```python
from build123d import *

# Parameters (mm, degrees)
F2_R     = 6.940355
F3_DEPTH = 279.4
F4_DEPTH = 25.4


with BuildPart() as f1:
    # F0 (on Front) → F1 (revolve)
    with BuildSketch(Plane.XZ):
        Polygon((0, -12.7), (0, 0), (53.81389, 53.949098), (49.866706, 57.886391), (-4.610259, 3.272552), (-12.603007, 2.86432), (-12.603007, -12.7), align=None)
    revolve(axis=Axis((-12.603007, 0, -4.91784), (0, 0, 1)))

    # F2 (on Top) → F3 (cut)
    with BuildSketch(Plane.XY):
        with Locations((-12.676277, 0)):
            Circle(F2_R)
    extrude(amount=-F3_DEPTH, mode=Mode.SUBTRACT)

    # F2 (on Top) → F4 (cut)
    with BuildSketch(Plane.XY):
        with Locations((-12.676277, 0)):
            Circle(F2_R)
    extrude(amount=F4_DEPTH, mode=Mode.SUBTRACT)


solid = f1.part
```
Check sheet for the modelled part. Datum: model origin and axes. Units: mm. Round coordinates to 2 decimals unless told otherwise and drop trailing zeros. Loops run counter-clockwise (first coordinate to the right, second up) from the corner with the lowest first, then second, coordinate; pieces in that order, holes last. Notation, with made-up numbers: (35, 71.25) -> (62, 71.25) arc R7 ccw to (62, 80.25) -> close; hole circle Ø1 at (51, 59). An arc over 180 degrees is marked (long way). Write item = value, one per line. Start each with the question number.
1) Release check for a two-part mould opening along Y. For faces 1 (the cylindrical face through (-0.961, -4.827, -6.261)), 2 (the flat face through (-18, -5, -12.7)), 3 (the conical face through (3.317, 5.013, 11.993)) record: released by +Y, released by -Y, zero draft, split by the parting line, or undercut.
2) Gauge pin test, flat ends, axial feed: pin 1 Ø8 at (x, y) = (4, -47.5) entering from +Z; pin 2 Ø8 at (x, z) = (-12, 49) entering from -Y; pin 3 Ø6 at (x, z) = (-24.5, -3.5) entering from -Y; pin 4 Ø6 at (x, z) = (14, 6) entering from +Y. Record the tip position at first contact, or that the pin passes through.
3) Sectioned sample at A-A, the plane y = 0. Record the cut outline in (x, z).
4) Thickness scan on probe 1 along X at (y, z) = (-16, 18.5); probe 2 along X at (y, z) = (13.5, 50.5); probe 3 along Y at (x, z) = (-41.5, 37.5). Record the ranges inside material, lowest first.
5) Sectioned sample at C-C, the plane z = 15.5. Record the cut outline in (x, y).
6) Sectioned sample at B-B, the plane z = 6. Record the cut outline in (x, y).
Results are:
q1.face_1 = split by the parting line
q1.face_2 = zero draft
q1.face_3 = undercut
q2.pin_1 = 49.71
q2.pin_2 = -65.47
q2.pin_3 = -8.93
q2.pin_4 = through
q3.outline = (-79.02, 53.95) -> (-25.21, 0) -> (-25.21, -12.7) -> (-19.62, -12.7) -> (-19.62, 3.22) -> (-20.6, 3.27) -> (-75.07, 57.89) -> close; (-5.74, -12.7) -> (0, -12.7) -> (0, 0) -> (53.81, 53.95) -> (49.87, 57.89) -> (-4.61, 3.27) -> (-5.74, 3.22) -> close
q4.probe_1 = -39.22 to -29.38, 4.17 to 14.01
q4.probe_2 = -74.12 to -66.03, 40.82 to 48.91
q4.probe_3 = -40.82 to -30.66, 30.66 to 40.82
q5.outline = circle Ø56.13 at (-12.6, 0); hole circle Ø40.38 at (-12.6, 0)
q6.outline = circle Ø37.18 at (-12.6, 0); hole circle Ø21.43 at (-12.6, 0)
